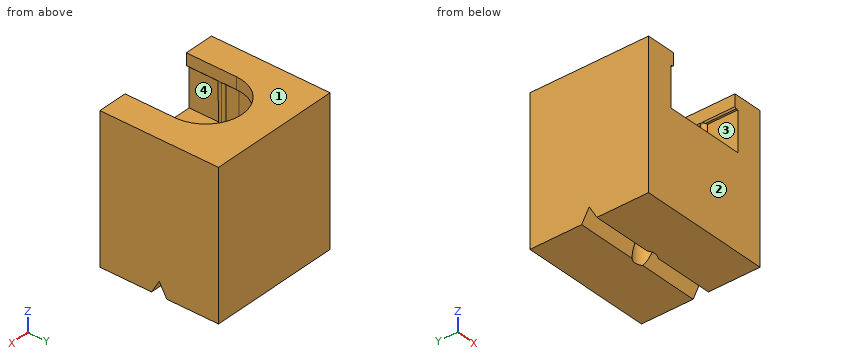
```python
from build123d import *

# Parameters (mm, degrees)
BOSS_EXTRUDE1_DEPTH = 4
SKETCH2_W           = 10
SKETCH2_H           = 9
BOSS_EXTRUDE2_DEPTH = 7
SKETCH3_R           = 0.75
CUT_EXTRUDE1_DEPTH  = 6
CUT_EXTRUDE3_REACH  = 15.273
BOSS_EXTRUDE3_START = -1
BOSS_EXTRUDE3_DEPTH = 1
CHAMFER1_SIZE       = 0.1


with BuildPart() as part:
    # Sketch1 → Boss-Extrude1 (new body)
    with BuildSketch(Plane.XY):
        with BuildLine():
            Line((-3, -3.786060838), (-3, -1.49999581))
            ThreePointArc((-3, -1.49999581), (-2.791987509, -1.388670983), (-2.769230655, -1.153842239))
            ThreePointArc((-2.769230655, -1.153842239), (-2.861324827, -1.041983319), (-3, -0.99999581))
            Line((-3, -0.99999581), (-3, 0))
            ThreePointArc((-3, 0), (0, 3), (3, 0))
            Line((3, 0), (3, -0.99999581))
            ThreePointArc((3, -0.99999581), (2.861324827, -1.041983319), (2.769230655, -1.153842239))
            ThreePointArc((2.769230655, -1.153842239), (2.791987509, -1.388670983), (3, -1.49999581))
            Line((3, -1.49999581), (3, -3.786060838))
            Line((3, -3.786060838), (5, -3.786060838))
            Line((5, -3.786060838), (5, 5.213939162))
            Line((5, 5.213939162), (-5, 5.213939162))
            Line((-5, 5.213939162), (-5, -3.786060838))
            Line((-5, -3.786060838), (-3, -3.786060838))
        make_face()
    extrude(amount=BOSS_EXTRUDE1_DEPTH)

    # Sketch2 → Boss-Extrude2 (add)
    with BuildSketch(Plane.XY):
        with Locations((0, 0.713939162)):
            Rectangle(SKETCH2_W, SKETCH2_H)
    extrude(amount=-BOSS_EXTRUDE2_DEPTH)

    # Sketch3 → Cut-Extrude1 (cut)
    with BuildSketch(Plane(origin=(0, 0, -7), x_dir=(-1, 0, 0), z_dir=(0, 0, -1))):
        with Locations((0, 0.713939162)):
            Circle(SKETCH3_R)
    extrude(amount=-CUT_EXTRUDE1_DEPTH, mode=Mode.SUBTRACT)

    # Cut-Extrude3: up to this face of the body (flat: up to its plane)
    cut_extrude3_end = Plane(part.part.faces().sort_by_distance((-5, 0.713939162, -1.5))[0])
    # Sketch4 → Cut-Extrude3 (cut, up to the picked face)
    with BuildSketch(Plane(origin=(5, 0, 0), x_dir=(0, 0, -1), z_dir=(1, 0, 0)), mode=Mode.PRIVATE) as cut_extrude3_sk1:
        Polygon((7.5, -0.152086242), (7.5, 1.579964565), (6, 0.713939162), align=None)
    cut_extrude3_tool1 = split(extrude(cut_extrude3_sk1.sketch, amount=-CUT_EXTRUDE3_REACH, mode=Mode.PRIVATE), bisect_by=cut_extrude3_end, keep=Keep.BOTH, mode=Mode.PRIVATE)
    add(cut_extrude3_tool1.solids().sort_by(Axis((5, 0.713939, -7), (-1, 0, 0)))[0], mode=Mode.SUBTRACT)

    # Sketch5 → Boss-Extrude3 (add)
    with BuildSketch(Plane.XY.offset(4).offset(BOSS_EXTRUDE3_START)):
        with BuildLine():
            ThreePointArc((3, 0), (0, 3), (-3, 0))
            Line((-3, 0), (-3, -3.786060838))
            Line((-3, -3.786060838), (-2.75, -3.786060838))
            Line((-2.75, -3.786060838), (-2.75, 0))
            ThreePointArc((-2.75, 0), (0, 2.75), (2.75, 0))
            Line((2.75, 0), (2.75, -3.786060838))
            Line((2.75, -3.786060838), (3, -3.786060838))
            Line((3, -3.786060838), (3, 0))
        make_face()
    extrude(amount=BOSS_EXTRUDE3_DEPTH)

    # Chamfer1
    # the kernel refuses this chamfer: 0.1 mm, written as the material it takes off along each edge
    with BuildSketch(Plane(origin=(2.75, -1.24999581, 3), x_dir=(-0.027495876610587302, 0, 0.9996219169112966), z_dir=(0, -1, 0))) as chamfer1_piece_1_section:
        Polygon((CHAMFER1_SIZE * 0.999621916911, -CHAMFER1_SIZE * 0.0274958766106), (-CHAMFER1_SIZE * 0.0274958766106, -CHAMFER1_SIZE * 0.999621916911), (0, 0), align=None)
    chamfer1_piece_1 = extrude(amount=2.793233327, mode=Mode.PRIVATE)
    chamfer1_piece_1 = chamfer1_piece_1 - Plane(origin=(3, -1.24999581, 3.033543391), x_dir=(0, 1, 0), z_dir=(0, 0, -1)) * Cylinder(0.25, 6, mode=Mode.PRIVATE)
    add(chamfer1_piece_1, mode=Mode.SUBTRACT)
    with BuildSketch(Plane(origin=(-2.75, -4.043229137, 3), x_dir=(-0.9996219169112966, 0, -0.027495876610587302), z_dir=(0, 1, 0))) as chamfer1_piece_2_section:
        Polygon((CHAMFER1_SIZE * 0.999621916911, CHAMFER1_SIZE * 0.0274958766106), (-CHAMFER1_SIZE * 0.0274958766106, CHAMFER1_SIZE * 0.999621916911), (0, 0), align=None)
    chamfer1_piece_2 = extrude(amount=2.793233327, mode=Mode.PRIVATE)
    chamfer1_piece_2 = chamfer1_piece_2 - Plane(origin=(-3, -1.24999581, 3.033543414), x_dir=(0, -1, 0), z_dir=(0, 0, -1)) * Cylinder(0.25, 6, mode=Mode.PRIVATE)
    add(chamfer1_piece_2, mode=Mode.SUBTRACT)
    with BuildSketch(Plane(origin=(2.75, 0, 3), x_dir=(-0.027495876610587302, 0, 0.9996219169112966), z_dir=(0, -1, 0))) as chamfer1_piece_3_section:
        Polygon((CHAMFER1_SIZE * 0.999621916911, -CHAMFER1_SIZE * 0.0274958766106), (-CHAMFER1_SIZE * 0.0274958766106, -CHAMFER1_SIZE * 0.999621916911), (0, 0), align=None)
    chamfer1_piece_3 = extrude(amount=1.24999581, mode=Mode.PRIVATE)
    chamfer1_piece_3 = chamfer1_piece_3 - Plane(origin=(3, -1.24999581, 3.033781207), x_dir=(0, 1, 0), z_dir=(0, 0, -1)) * Cylinder(0.25, 3, mode=Mode.PRIVATE)
    add(chamfer1_piece_3, mode=Mode.SUBTRACT)
    with BuildSketch(Plane(origin=(0, 0, 3), x_dir=(-1, 0, 0), z_dir=(0, -1, 0))) as chamfer1_piece_4:
        Polygon((2.75, -CHAMFER1_SIZE), (2.75 + CHAMFER1_SIZE, 0), (2.75, 0), align=None)
    revolve(axis=Axis((0, 0, 3), (0, 0, -1)), revolution_arc=180, mode=Mode.SUBTRACT)
    with BuildSketch(Plane(origin=(-2.75, -1.24999581, 3), x_dir=(-0.9996219169112966, 0, -0.027495876610587302), z_dir=(0, 1, 0))) as chamfer1_piece_5_section:
        Polygon((CHAMFER1_SIZE * 0.999621916911, CHAMFER1_SIZE * 0.0274958766106), (-CHAMFER1_SIZE * 0.0274958766106, CHAMFER1_SIZE * 0.999621916911), (0, 0), align=None)
    chamfer1_piece_5 = extrude(amount=1.24999581, mode=Mode.PRIVATE)
    chamfer1_piece_5 = chamfer1_piece_5 - Plane(origin=(-3, -1.24999581, 3.033781195), x_dir=(0, -1, 0), z_dir=(0, 0, -1)) * Cylinder(0.25, 3, mode=Mode.PRIVATE)
    add(chamfer1_piece_5, mode=Mode.SUBTRACT)


solid = part.part
```
Geometry check sheet. Reference: the model listing, model coordinates, mm. Face numbers are marked on the shaded views. Round coordinates to 2 decimals unless told otherwise and drop trailing zeros. Order: outer loops, then holes, each group sorted by start corner. A loop starts at its lowest first (then second) coordinate and runs counter-clockwise, first axis right, second up. Notation, with made-up numbers: (87, 38) - (122, 38) arc R7 ccw to (122, 51) - close; hole circle Ø3 at (-21, -9.5). An arc over 180 degrees is marked (long way). Use a Markdown table: item, result. Add a question column.
1) Mould release check, pull along Z, two halves, no side actions. Record for the marked faces 1, 2, 3 and 4: released by +Z, released by -Z, zero draft, split by the parting line, or undercut.
2) Thickness scan on line 1 along X through (y, z) = (-1.25, 0.25); line 2 along Y through (x, z) = (0, -3.8). Record the ranges inside material, lowest first.
3) Section check C-C (z = -5.75). Record the cut outline in (x, y), then the cut area to 3 significant figures.
4) Gauge pin test, flat end, axial feed: P1, Ø1.4, axis at x = 0, y = 0.71, coming from the +Z side. Record the tip position at first contact, or that the pin passes through.
5) Section check A-A (x = 0). Record the cut outline in (y, z).
6) Section check B-B (z = 1). Record the cut outline in (x, y), then the cut area to 3 significant figures.
Established:
| question | item | result |
|---|---|---|
| 1 | face 1 | released by +Z |
| 1 | face 2 | zero draft |
| 1 | face 3 | undercut |
| 1 | face 4 | undercut |
| 2 | line 1 | -5 to -2.75, 2.75 to 5 |
| 2 | line 2 | -3.79 to -0.04, 1.46 to 5.21 |
| 3 | outline | (-5, -3.79) - (5, -3.79) - (5, 5.21) - (-5, 5.21) - close; hole circle Ø1.5 at (0, 0.71) |
| 3 | area | 88.2 mm2 |
| 4 | P1 | z = 0 |
| 5 | outline | (-3.79, -7) - (-0.04, -7) - (-0.04, -1) - (1.46, -1) - (1.46, -7) - (5.21, -7) - (5.21, 4) - (2.75, 4) - (2.75, 3.1) - (2.85, 3) - (3, 3) - (3, 0) - (-3.79, 0) - close |
| 6 | outline | (-5, -3.79) - (-3, -3.79) - (-3, -1.5) arc R0.25 ccw to (-3, -1) - (-3, 0) arc R3 cw to (3, 0) - (3, -1) arc R0.25 ccw to (3, -1.5) - (3, -3.79) - (5, -3.79) - (5, 5.21) - (-5, 5.21) - close |
| 6 | area | 53.3 mm2 |
